```python
from build123d import *

# Parameters (mm, degrees)
BOSS_EXTRUDE1_DEPTH = 5
CUT_EXTRUDE1_DEPTH  = 0.7
SKETCH7_W           = 168.55
SKETCH7_H           = 99.71
CUT_EXTRUDE2_DEPTH  = 166.54571941
SKETCH8_R           = 11.1025
CUT_EXTRUDE3_DEPTH  = 166.54571941
CHAMFER1_SIZE       = 0.365
SKETCH58_R          = 6
CUT_EXTRUDE4_DEPTH  = 166.54571941
SKETCH59_R          = 9.5
CUT_EXTRUDE5_DEPTH  = 166.54571941


# Read off the part's stored shape, not the designer's step: Cut-Sweep1, Cut-Sweep2
with BuildPart() as part:
    # Sketch1 → Boss-Extrude1 (new body)
    with BuildSketch(Plane.XY):
        with BuildLine():
            Line((-130, 69.8597539), (130, 69.8597539))
            ThreePointArc((130, 69.8597539), (144.142135624, 64.001889524), (150, 49.8597539))
            Line((150, 49.8597539), (150, -49.8597539))
            ThreePointArc((150, -49.8597539), (144.142135624, -64.001889524), (130, -69.8597539))
            Line((130, -69.8597539), (-130, -69.8597539))
            ThreePointArc((-130, -69.8597539), (-144.142135624, -64.001889524), (-150, -49.8597539))
            Line((-150, -49.8597539), (-150, 49.8597539))
            ThreePointArc((-150, 49.8597539), (-144.142135624, 64.001889524), (-130, 69.8597539))
        make_face()
    extrude(amount=BOSS_EXTRUDE1_DEPTH)

    # Sketch5 → Cut-Extrude1 (cut)
    with BuildSketch(Plane.XY):
        with BuildLine():
            Line((-94.3997539, 52.3802461), (-94.3997539, -51.8597539))
            ThreePointArc((-94.3997539, -51.8597539), (-92.05660815, -57.51660815), (-86.3997539, -59.8597539))
            Line((-86.3997539, -59.8597539), (86.9202461, -59.8597539))
            ThreePointArc((86.9202461, -59.8597539), (92.577100349, -57.51660815), (94.9202461, -51.8597539))
            Line((94.9202461, -51.8597539), (94.9202461, 52.3802461))
            ThreePointArc((94.9202461, 52.3802461), (92.577100349, 58.037100349), (86.9202461, 60.3802461))
            Line((86.9202461, 60.3802461), (-86.3997539, 60.3802461))
            ThreePointArc((-86.3997539, 60.3802461), (-92.05660815, 58.037100349), (-94.3997539, 52.3802461))
        make_face()
    extrude(amount=CUT_EXTRUDE1_DEPTH, mode=Mode.SUBTRACT)

    # Sketch7 → Cut-Extrude2 (cut, through all)
    with BuildSketch(Plane.XY):
        Rectangle(SKETCH7_W, SKETCH7_H)
    extrude(amount=CUT_EXTRUDE2_DEPTH, mode=Mode.SUBTRACT)

    # Sketch8 → Cut-Extrude3 (cut, through all)
    with BuildSketch(Plane.XY.offset(5)):
        with Locations((-117.1375, 40)):
            Circle(SKETCH8_R)
        with Locations(Location((117.1375, 40, 0), (0, 0, 180))):
            Circle(SKETCH8_R)
    extrude(amount=-CUT_EXTRUDE3_DEPTH, mode=Mode.SUBTRACT)

    # Chamfer1
    chamfer1_edges = [part.edges().sort_by_distance(p)[0] for p in [
        (-128.24, 40, 0),
        (128.24, 40, 0),
    ]]
    chamfer(chamfer1_edges, length=CHAMFER1_SIZE)

    # Cut-Sweep1 outline → Cut-Sweep1 (revolve, cut)
    with BuildSketch(Plane(origin=(-117.1375, 40, 0), x_dir=(1, 0, 0), z_dir=(0, -1, 0))):
        with BuildLine():
            Line((11.1025, 5), (11.1025, 1.5))
            ThreePointArc((11.1025, 1.5), (13.577373734, 2.525126266), (14.6025, 5))
            Line((14.6025, 5), (11.1025, 5))
        make_face()
    revolve(axis=Axis((-117.1375, 40, 0), (0, 0, 1)), mode=Mode.SUBTRACT)

    # Cut-Sweep2 outline → Cut-Sweep2 (revolve, cut)
    with BuildSketch(Plane(origin=(117.1375, 40, 0), x_dir=(1, 0, 0), z_dir=(0, -1, 0))):
        with BuildLine():
            Line((11.1025, 5), (11.1025, 1.5))
            ThreePointArc((11.1025, 1.5), (13.577373734, 2.525126266), (14.6025, 5))
            Line((14.6025, 5), (11.1025, 5))
        make_face()
    revolve(axis=Axis((117.1375, 40, 0), (0, 0, 1)), mode=Mode.SUBTRACT)

    # Sketch58 → Cut-Extrude4 (cut, through all)
    with BuildSketch(Plane(origin=(0, 0, 0), x_dir=(-1, 0, 0), z_dir=(0, 0, -1))):
        with Locations((-125, 13)):
            Circle(SKETCH58_R)
        with Locations((-112, 0)):
            Circle(SKETCH58_R)
        with Locations((-125, -13)):
            Circle(SKETCH58_R)
        with Locations((-137.5, 0)):
            Circle(SKETCH58_R)
    extrude(amount=-CUT_EXTRUDE4_DEPTH, mode=Mode.SUBTRACT)

    # Sketch59 → Cut-Extrude5 (cut, through all)
    with BuildSketch(Plane(origin=(0, 0, 0), x_dir=(-1, 0, 0), z_dir=(0, 0, -1))):
        with Locations((125, -49.8597539)):
            Circle(SKETCH59_R)
    extrude(amount=-CUT_EXTRUDE5_DEPTH, mode=Mode.SUBTRACT)


solid = part.part
```
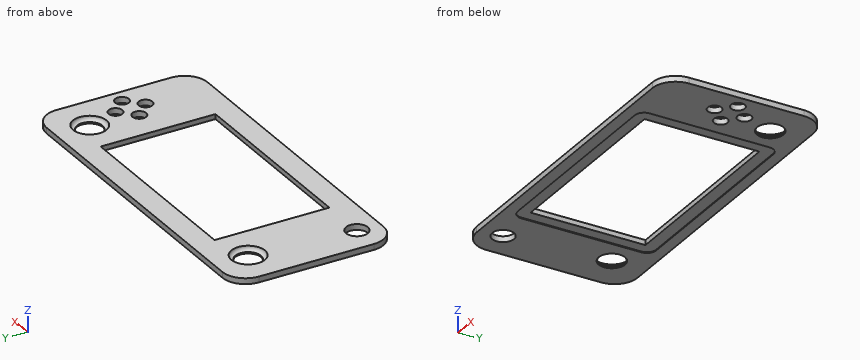
Can you work these out from the model? Positions are in its coordinate system, mm. Coordinates: 2 decimals unless noted, no trailing zeros. Loops run counter-clockwise (first coordinate to the right, second up) from the corner with the lowest first, then second, coordinate; pieces in that order, holes last.
1) Imagine slicing it at A-A on y = 13. List the corners of the cut face in (x, z) for me (3 decimals), plus the area to 3 significant figures.
2) Imagine slicing it at D-D on y = -16. List the corners of the cut face in (x, z) for me (3 decimals).
3) Imagine slicing it at B-B on x = -26.5. List the corners of the cut face in (y, z) for me (3 decimals).
4) Imagine slicing it at C-C on z = 4. State how many separate pieces and enclosed holes the cut face has, plus the area to 3 significant figures.
5) I need wall thicknesses on probe 1 along Y at (x, z) = (-82.5, 2.85) (3 decimals); probe 2 along X at (y, z) = (-4.5, 4.25) (3 decimals); probe 3 along X at (y, z) = (-25, 3.7) (3 decimals). Which ranges of each line are inside material? Lowest first, please.
Completed:
1. outline: (-150, 0) - (-94.4, 0) - (-94.4, 0.7) - (-84.275, 0.7) - (-84.275, 5) - (-150, 5) - close; (84.275, 0.7) - (94.92, 0.7) - (94.92, 0) - (119, 0) - (119, 5) - (84.275, 5) - close; (131, 0) - (150, 0) - (150, 5) - (131, 5) - close
1. area: 583 mm2
2. outline: (-150, 0) - (-94.4, 0) - (-94.4, 0.7) - (-84.275, 0.7) - (-84.275, 5) - (-150, 5) - close; (84.275, 0.7) - (94.92, 0.7) - (94.92, 0) - (119.804, 0) - (119.804, 5) - (84.275, 5) - close; (130.196, 0) - (150, 0) - (150, 5) - (130.196, 5) - close
3. outline: (-69.86, 0) - (-59.86, 0) - (-59.86, 0.7) - (-49.855, 0.7) - (-49.855, 5) - (-69.86, 5) - close; (49.855, 0.7) - (60.38, 0.7) - (60.38, 0) - (69.86, 0) - (69.86, 5) - (49.855, 5) - close
4. separate pieces: 1
4. enclosed holes: 8
4. area: 22,700 mm2
5. probe 1: y = -69.86 to -49.855, 49.855 to 69.86
5. probe 2: x = -150 to -84.275, 84.275 to 108.031, 115.969 to 133.531, 141.469 to 150
5. probe 3: x = -150 to -84.275, 84.275 to 150
